Work out the finished part from the listing and answer in its coordinate system (mm). Face numbers are marked on the shaded views. A direction names the side the tool comes from. Coordinates: 2 decimals unless noted, no trailing zeros. Loops run counter-clockwise (first coordinate to the right, second up) from the corner with the lowest first, then second, coordinate; pieces in that order, holes last. Notation, with made-up numbers: (25.5, 62) -> (38.5, 62) arc R10 ccw to (38.5, 75) -> close; hole circle Ø10 at (-37, 63). An arc over 180 degrees is marked (long way). One line per question, with ' | ' between items.
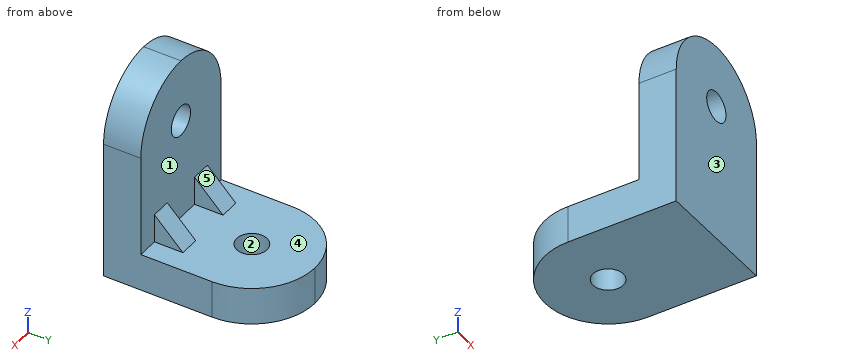
```python
from build123d import *

# Parameters (mm, degrees)
F0_R     = 1.5
F2_DEPTH = 3.7
F1_R     = 1.5
F3_DEPTH = 3.7
F6_W     = 2
F6_H     = 4
F7_DEPTH = 4


with BuildPart() as f2:
    # F0 (on Front) → F2 (new body)
    with BuildSketch(Plane.XZ):
        with BuildLine():
            Line((0, 13.75), (0, 0))
            Line((0, 0), (12.5, 0))
            Line((12.5, 0), (12.5, 13.75))
            ThreePointArc((12.5, 13.75), (10.6694173824, 18.1694173824), (6.25, 20))
            ThreePointArc((6.25, 20), (1.8305826176, 18.1694173824), (0, 13.75))
        make_face()
        with Locations((6.25, 13.75)):
            Circle(F0_R, mode=Mode.SUBTRACT)
    extrude(amount=-F2_DEPTH)

    # F1 (on Top) → F3 (join)
    with BuildSketch(Plane.XY):
        with BuildLine():
            Line((0, 10.75), (0, 0))
            Line((0, 0), (12.5, 0))
            Line((12.5, 0), (12.5, 10.75))
            ThreePointArc((12.5, 10.75), (10.6694173824, 15.1694173824), (6.25, 17))
            ThreePointArc((6.25, 17), (1.8305826176, 15.1694173824), (0, 10.75))
        make_face()
        with Locations((6.25, 10.75)):
            Circle(F1_R, mode=Mode.SUBTRACT)
    extrude(amount=F3_DEPTH)

    # F6 (on face) → F7 (join)
    with BuildSketch(Plane(origin=(0, 5.1142135624, 5.1142135624), x_dir=(1, 0, 0), z_dir=(0, -0.7071067812, -0.7071067812))):
        with Locations((9.375, 0)):
            Rectangle(F6_W, F6_H)
        with Locations((3.125, 0)):
            Rectangle(F6_W, F6_H)
    extrude(amount=F7_DEPTH)


solid = f2.part
```
1) The mould has two halves that part along Y. Classify the marked faces 1, 2 and 3: released by +Y, released by -Y, zero draft, split by the parting line, or undercut.
Check values:
face 1: released by +Y | face 2: undercut | face 3: released by -Y
2) Find section D-D (y = 1.75). Write down the section's boundary in (x, z).
Check values:
outline: (0, 0) -> (12.5, 0) -> (12.5, 13.75) arc R6.25 ccw to (0, 13.75) -> close; hole circle Ø3 at (6.25, 13.75)
3) Flat-ended cylindrical pins translate along their axes: pin 1 (6 mm diameter, centred on x = 8.5, z = 8, fed in from +Y); pin 2 (8 mm diameter, centred on y = 7.5, z = 12.5, fed in from -X); pin 3 (4 mm diameter, centred on x = 6.25, y = 10.75, fed in from +Z); pin 4 (2.5 mm diameter, centred on y = 5, z = 5, fed in from +X) (3 decimals). Find the tip coordinate at first contact, or state that the pin passes through.
Check values:
pin 1: stops at y = 5.23 | pin 2: stops at x = 0 | pin 3: stops at z = 3.7 | pin 4: stops at x = 10.375
4) Find section A-A (x = 7.5). Write down the section's boundary in (y, z), plus the area to 3 significant figures.
Check values:
outline: (0, 0) -> (9.92, 0) -> (9.92, 3.7) -> (3.7, 3.7) -> (3.7, 12.92) -> (0, 12.92) -> close; (0, 14.58) -> (3.7, 14.58) -> (3.7, 19.87) -> (0, 19.87) -> close; (11.58, 0) -> (16.87, 0) -> (16.87, 3.7) -> (11.58, 3.7) -> close | area: 110 mm^2
5) Find section C-C (z = 2.5). Write down the section's boundary in (x, y), plus the area to 3 significant figures.
Check values:
outline: (0, 0) -> (12.5, 0) -> (12.5, 10.75) arc R6.25 ccw to (0, 10.75) -> close; hole circle Ø3 at (6.25, 10.75) | area: 189 mm^2
6) Find section B-B (y = 11.5). Write down the section's boundary in (x, z), plus the area to 3 significant figures.
Check values:
outline: (0.05, 0) -> (4.95, 0) -> (4.95, 3.7) -> (0.05, 3.7) -> close; (7.55, 0) -> (12.45, 0) -> (12.45, 3.7) -> (7.55, 3.7) -> close | area: 36.3 mm^2
7) Find the intervals of material crossed by line 1 along Y through (x, z) = (6.25, 1.8); line 2 along Z through (x, y) = (6.25, 1.8); line 3 along Z through (x, y) = (6.75, 12.75), in increasing order.
Check values:
line 1: y = 0 to 9.25, 12.25 to 17 | line 2: z = 0 to 12.25, 15.25 to 20 | line 3: z = 0 to 3.7
8) For the marked faces 4 and 5, determine the directions among +Z, -Z, +X, -X, +Y, -Y from which every point of the face is accessible in a straight line to the end or side of a thin tool.
Check values:
face 4: +Z, +Y | face 5: +Z, +X, -X, +Y
